Could you check a few things on this model? Use its own coordinates, in mm. Round coordinates to 2 decimals unless told otherwise and drop trailing zeros. Write each loop counter-clockwise with the first axis right and the second up, starting at its lowest first coordinate (ties: lowest second). Pieces come first, ordered by that corner, then holes. Notation, with made-up numbers: (-2, 7) - (50, 7) arc R17 ccw to (50, 38) - close; hole circle Ø7 at (75, -5). An arc over 180 degrees is marked (long way). Write each question's results on one line, items separated by ' | '. Start each with the question number.
(1) Imagine slicing it at A-A on z = -10. Write out the boundary of the cut face in (x, y) (3 decimals), then the cut area to 3 significant figures.
(2) Please list where these lines run through material, in increasing order: line 1 (X direction, y = 5, z = -8); line 2 (X direction, y = -6, z = 12.5); line 3 (Z direction, x = -23, y = -1). Write a range as [from, to].
(3) Imagine slicing it at C-C on z = 15.5. Write out the boundary of the cut face in (x, y) (3 decimals).
(4) Imagine slicing it at D-D on x = 0. Write out the boundary of the cut face in (y, z) (3 decimals).
(5) Imagine slicing it at B-B on y = 6.75. Write out the boundary of the cut face in (x, z) (3 decimals), then the cut area to 3 significant figures.
(6) Thinking about a two-plate mould opening in Z: for faces 1 (the flat face through (-31.75, 0, -9)), 2 (the cylindrical face through (-21.486, 0.133, -9.024)), 3 (the flat face through (0, 0, -19.05)), 4 (the cylindrical face through (27.351, 0.133, -9.024)), which applies, +Z half, -Z half, draft (parallel to the pull), parting line (faces both ways), or undercut?
(7) For P1, Ø3, axis at x = 9, y = 1.5, coming from the +Z side; P2, Ø3, axis at y = 0, z = 10, coming from the +X side; P3, Ø6, axis at y = -5.5, z = 12, coming from the -X side; P4, Ø8, axis at x = -24.5, y = -7, coming from the +Z side, each with a flat end and sliding along its axis, tell me the tip position at first contact or that it passes through.
```python
from build123d import *

# Parameters (mm, degrees)
F0_R     = 3.175
F1_DEPTH = 9.525


with BuildPart() as f1:
    # F0 (on Front) → F1 (new body, symmetric)
    with BuildSketch(Plane.XZ):
        with BuildLine():
            Line((-9.525, 19.05), (-17.036222, 19.05))
            Line((-17.036222, 19.05), (-31.75, 0))
            Line((-31.75, 0), (-31.75, -19.05))
            Line((-31.75, -19.05), (31.75, -19.05))
            Line((31.75, -19.05), (31.75, 0))
            Line((31.75, 0), (17.036222, 19.05))
            Line((17.036222, 19.05), (9.525, 19.05))
            ThreePointArc((9.525, 19.05), (0, 9.525), (-9.525, 19.05))
        make_face()
        with Locations((-24.418587, -7.808267)):
            Circle(F0_R, mode=Mode.SUBTRACT)
        with Locations((24.418587, -7.808267)):
            Circle(F0_R, mode=Mode.SUBTRACT)
    extrude(amount=F1_DEPTH, both=True)


with BuildPart() as f2_1:
    # F2: copy of F1
    add(f1.part)


solid = f1.part
```
Response:
1) outline: (-31.75, -9.525) - (-26.716, -9.525) - (-26.716, 9.525) - (-31.75, 9.525) - close; (-22.121, -9.525) - (22.121, -9.525) - (22.121, 9.525) - (-22.121, 9.525) - close; (26.716, -9.525) - (31.75, -9.525) - (31.75, 9.525) - (26.716, 9.525) - close | area: 1,030 mm²
2) line 1: [-31.75, -27.59], [-21.25, 21.25], [27.59, 31.75] | line 2: [-22.1, -6.92], [6.92, 22.1] | line 3: [-19.05, -10.65], [-4.97, 11.33]
3) outline: (-19.778, -9.525) - (-8.839, -9.525) - (-8.839, 9.525) - (-19.778, 9.525) - close; (8.839, -9.525) - (19.778, -9.525) - (19.778, 9.525) - (8.839, 9.525) - close
4) outline: (-9.525, -19.05) - (9.525, -19.05) - (9.525, 9.525) - (-9.525, 9.525) - close
5) outline: (-31.75, -19.05) - (31.75, -19.05) - (31.75, 0) - (17.036, 19.05) - (9.525, 19.05) arc R9.525 cw to (-9.525, 19.05) - (-17.036, 19.05) - (-31.75, 0) - close; hole circle Ø6.35 at (-24.419, -7.808); hole circle Ø6.35 at (24.419, -7.808) | area: 1,930 mm²
6) face 1: draft | face 2: undercut | face 3: -Z half | face 4: undercut
7) P1: z = 19.05 | P2: x = 25.18 | P3: x = -24.8 | P4: z = 14.57
